Read the model definition and answer for the solid it produces. Units are mm, in the model's axes. Face numbers are marked on the shaded views. A direction names the side the tool comes from. Round coordinates to 2 decimals unless told otherwise and drop trailing zeros. Loops run counter-clockwise (first coordinate to the right, second up) from the corner with the lowest first, then second, coordinate; pieces in that order, holes last. Notation, with made-up numbers: M -32.75,69 L 25.25,69 A21 ccw 25.25,92 Z; hole C 60,37 d10. An arc over 180 degrees is marked long. Write each question's results on one line, items separated by ' | '.
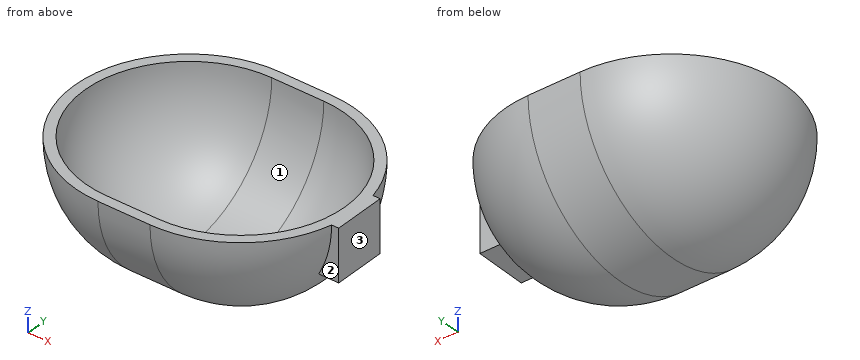
from build123d import *

# Parameters (mm, degrees)
REVOLVE1_ANGLE           = 180
SHELL1_T                 = -50
BOSS_EXTRUDE2_REACH      = 1600.609
BOSS_EXTRUDE2_END_RADIUS = 558
SKETCH5_W                = 254
SKETCH5_H                = 254


with BuildPart() as part:
    # Sketch2 → Revolve1 (revolve)
    with BuildSketch(Plane.XY):
        with BuildLine():
            Line((-279, 0), (279, 0))
            Line((279, 0), (533, 0))
            Line((533, 0), (1091, 0))
            ThreePointArc((1091, 0), (927.565583902, -394.565583902), (533, -558))
            Line((533, -558), (279, -558))
            ThreePointArc((279, -558), (-115.565583902, -394.565583902), (-279, 0))
        make_face()
    revolve(axis=Axis((533, 0, 0), (1, 0, 0)), revolution_arc=REVOLVE1_ANGLE)

    # Shell1
    shell1_openings = [part.faces().sort_by_distance(p)[0] for p in [
        (406, 0, 0),
    ]]
    offset(amount=SHELL1_T, openings=shell1_openings)

    # Boss-Extrude2: up to this sphere (the profile starts outside it)
    boss_extrude2_end = Location((533, 0, 0)) * Sphere(BOSS_EXTRUDE2_END_RADIUS, mode=Mode.PRIVATE)
    # Sketch5 → Boss-Extrude2 (add, up to the surface)
    with BuildSketch(Plane(origin=(1111.26, 0, 0), x_dir=(0, 0, -1), z_dir=(1, 0, 0)), mode=Mode.PRIVATE) as boss_extrude2_sk1:
        with Locations((127, 0)):
            Rectangle(SKETCH5_W, SKETCH5_H)
    boss_extrude2_tool1 = extrude(boss_extrude2_sk1.sketch, amount=-BOSS_EXTRUDE2_REACH, mode=Mode.PRIVATE) - boss_extrude2_end
    add(boss_extrude2_tool1.solids().sort_by_distance((1111.26, 0, -127))[0])


solid = part.part
Item 1: For the marked faces 1, 2 and 3, determine the directions among +Z, -Z, +X, -X, +Y, -Y from which every point of the face is accessible in a straight line to the end or side of a thin tool.
Outcome:
face 1: +Z | face 2: -Z, +X, -Y | face 3: +Z, -Z, +X, +Y, -Y
Item 2: Straight lines are drawn through the part: line 1 (Y direction, x = -155, z = -160); line 2 (Y direction, x = 794, z = -25); line 3 (X direction, y = 369.5, z = -314). For each, find the intervals that lie inside material, in ascending order.
Outcome:
line 1: y = -312.1 to -210.02, 210.02 to 312.1 | line 2: y = -492.56 to -435.11, 435.11 to 492.56 | line 3: x = 2.89 to 127.55, 684.45 to 809.11
Item 3: The part is cut by section B-B (y = 0). Determine the outline of the cut face in (x, z).
Outcome:
outline: M -279,0 A558 ccw 279,-558 L 533,-558 A558 ccw 1029.84,-254 L 1111.26,-254 L 1111.26,0 L 1041,0 A508 cw 533,-508 L 279,-508 A508 cw -229,0 Z
Item 4: The part is cut by section D-D (x = 721.5). Determine the outline of the cut face in (y, z), plus the area to 3 significant figures.
Outcome:
outline: M -525.2,0 A525.2 ccw 525.2,0 L 471.73,0 A471.73 cw -471.73,0 Z | area: 83,700 mm2
Item 5: The part is cut by section A-A (z = -97). Determine the outline of the cut face in (x, y).
Outcome:
outline: M 279,-549.5 L 533,-549.5 A549.5 ccw 1067.63,-127 L 1111.26,-127 L 1111.26,127 L 1067.63,127 A549.5 ccw 533,549.5 L 279,549.5 A549.5 ccw Z; hole M 279,-498.65 L 533,-498.65 A498.65 ccw 533,498.65 L 279,498.65 A498.65 ccw Z
Item 6: Flat-ended cylindrical pins translate along their axes: pin 1 (4 mm diameter, centred on y = 188, z = -353.5, fed in from -X); pin 2 (2 mm diameter, centred on y = -116.5, z = -444.5, fed in from +X); pin 3 (5 mm diameter, centred on x = 237.5, y = -398.5, fed in from +Z). Find the tip coordinate at first contact, or state that the pin passes through.
Outcome:
pin 1: stops at x = -111.71 | pin 2: stops at x = 851.01 | pin 3: stops at z = -309.08
Item 7: The part is cut by section C-C (z = -387). Determine the outline of the cut face in (x, y).
Outcome:
outline: M 279,-401.99 L 533,-401.99 A401.99 ccw 533,401.99 L 279,401.99 A401.99 ccw Z; hole M 279,-329.08 L 533,-329.08 A329.08 ccw 533,329.08 L 279,329.08 A329.08 ccw Z
